CAD build for the part. Positions are in the model's coordinates, mm. A direction names the side the tool comes from. Coordinates: 2 decimals unless noted, no trailing zeros. Loops run counter-clockwise (first coordinate to the right, second up) from the corner with the lowest first, then second, coordinate; pieces in that order, holes last. Notation, with made-up numbers: (18, 83.5) -> (63, 83.5) arc R36 ccw to (63, 121.5) -> close; hole circle Ø1 at (40, -38.75). An arc over 180 degrees is marked (long way). Return JSON: item names as keys, results as strings. Group by question number.
(1) Tool access for faces 4 (the face through (-8.116, -2.521, -4.541)), 5 (the face through (-8.021, -0.014, -9.833)), 6 (the face through (-7, 4, -8.25)): list every direction of +Z, -Z, +X, -X, +Y, -Y with a clear straight run to the whole face (end or side of a thin tool).
(2) Saw through at D-D on y = -2.75. Write the cut outline in (x, z).
(3) Saw through at A-A on y = -4.5. Write the cut outline in (x, z).
(4) Flat gauge pins, fed straight in: pin 1 Ø1.6 at (y, z) = (4.5, -1.5) entering from -X; pin 2 Ø8 at (x, y) = (9.5, -3) entering from -Z; pin 3 Ø1 at (y, z) = (-7.5, -17) entering from +X. Where does each tip first touch, or does it go through?
(5) Saw through at C-C on x = 14. Write the cut outline in (y, z), then the cut area to 3 significant figures.
(6) Probe L1, parallel to Y at x = -8.75, z = -10.75; L2, parallel to Z at x = -3, y = -1.5; L3, parallel to Y at x = -9.5, z = -5.5. List the from-to ranges inside material, lowest first.
(7) Saw through at B-B on y = 1.5. Write the cut outline in (x, z), then the cut area to 3 significant figures.
(8) Mould opens along Y. For faces 1 (the face through (-6, 3, -18)), 2 (the face through (-8.021, -5.014, -9.833)), 3 (the face through (3, 5, -9)) say: pulls with the +Y half, pulls with the -Y half, needs draft (parallel to the pull), parting line crosses it, or undercut.
```python
from build123d import *
from build123d.topology import SkipClean

# Parameters (mm, degrees)
SKETCH1_R           = 1.5
BOSS_EXTRUDE1_DEPTH = 5
BOSS_EXTRUDE2_START = 10
SKETCH2_R           = 1.5
BOSS_EXTRUDE2_DEPTH = 10
CUT_EXTRUDE1_DEPTH  = 2
SKETCH4_OUTSIDE_W   = 39.104
SKETCH4_OUTSIDE_H   = 31.904
SKETCH4_OUTSIDE_R   = 4
CUT_EXTRUDE2_DEPTH  = 2
FILLET4_R           = 7
CUT_EXTRUDE5_START  = -9
CUT_EXTRUDE5_DEPTH  = 7
CUT_EXTRUDE7_START  = 2
CUT_EXTRUDE7_DEPTH  = 2
LPATTERN1_COUNT     = 2
LPATTERN1_PITCH     = 5
CUT_EXTRUDE9_START  = -2
CUT_EXTRUDE9_DEPTH  = 2
LPATTERN2_COUNT     = 2
LPATTERN2_PITCH     = 5
FILLET5_START       = -6
FILLET5_DEPTH       = 2
FILLET5_START_2     = -1
FILLET5_2_DEPTH     = 1


with BuildPart() as part:
    # Sketch1 → Boss-Extrude1 (new body)
    with BuildSketch(Plane(origin=(0, 0, 0), x_dir=(1, 0, 0), z_dir=(0, 1, 0))):
        with BuildLine():
            Line((-12, 14), (-12, 22))
            Line((-12, 22), (-6, 22))
            Line((-6, 22), (-6, 14))
            Line((-6, 14), (0.894304297, 14))
            Line((0.894304297, 14), (6.85307226, 9))
            Line((6.85307226, 9), (11.887670047, 15))
            Line((11.887670047, 15), (15.887670047, 15))
            Line((15.887670047, 15), (17.2, 0))
            Line((17.2, 0), (-3, 0))
            ThreePointArc((-3, 0), (-4.264911064, 0.205266808), (-5.4, 0.8))
            ThreePointArc((-5.4, 0.8), (-10.258048651, 6.620975674), (-12, 14))
        make_face()
        with Locations(Location((-3, 4, 0), (0, 0, 270))):
            Circle(SKETCH1_R, mode=Mode.SUBTRACT)
    extrude(amount=BOSS_EXTRUDE1_DEPTH)

    # Sketch2 → Boss-Extrude2 (add)
    with SkipClean():  # the faces are left unmerged after this step: merging them gives an invalid solid
        with BuildSketch(Plane.XZ.offset(BOSS_EXTRUDE2_START)):
            with BuildLine():
                Line((-12, -14), (-12, -22))
                Line((-12, -22), (-6, -22))
                Line((-6, -22), (-6, -8))
                Line((-6, -8), (-3, -8))
                ThreePointArc((-3, -8), (1, -4), (-3, 0))
                ThreePointArc((-3, 0), (-4.264911064, -0.205266808), (-5.4, -0.8))
                ThreePointArc((-5.4, -0.8), (-10.258048651, -6.620975674), (-12, -14))
            make_face()
            with Locations(Location((-3, -4, 0), (0, 0, 270))):
                Circle(SKETCH2_R, mode=Mode.SUBTRACT)
        extrude(amount=-BOSS_EXTRUDE2_DEPTH)

    # Sketch3 → Cut-Extrude1 (cut)
    with SkipClean():  # the faces are left unmerged after this step: merging them gives an invalid solid
        with BuildSketch(Plane(origin=(0, 5, 0), x_dir=(1, 0, 0), z_dir=(0, 1, 0))):
            with BuildLine():
                Line((1.25, 4), (1.25, 0))
                Line((1.25, 0), (-10.965687828, 0))
                Line((-10.965687828, 0), (-10.965687828, 8.25))
                Line((-10.965687828, 8.25), (-3, 8.25))
                ThreePointArc((-3, 8.25), (0.00520382, 7.00520382), (1.25, 4))
            make_face()
        extrude(amount=-CUT_EXTRUDE1_DEPTH, mode=Mode.SUBTRACT)

    # Sketch4 outside → Cut-Extrude2 (cut)
    with SkipClean():  # the faces are left unmerged after this step: merging them gives an invalid solid
        with BuildSketch(Plane.XZ.offset(10)):
            with Locations((2.6, -11)):
                Rectangle(SKETCH4_OUTSIDE_W, SKETCH4_OUTSIDE_H)
            with Locations(Location((-3, -4, 0), (0, 0, 270))):
                Circle(SKETCH4_OUTSIDE_R, mode=Mode.SUBTRACT)
        extrude(amount=-CUT_EXTRUDE2_DEPTH, mode=Mode.SUBTRACT)

    # Fillet4
    # the kernel refuses this fillet: 7 mm, written as the material it adds along each edge
    with BuildSketch(Plane(origin=(-6, -8, -8), x_dir=(0, 0, -1), z_dir=(0, 1, 0))) as fillet4_piece_1:
        with BuildLine():
            CenterArc((5.744562647, -7), FILLET4_R, 90, 55.150095421)
            Line((0, -3), (0, 0))
            Line((0, 0), (5.744562647, 0))
        make_face()
    extrude(amount=8)

    # Sketch8 → Cut-Extrude5 (cut)
    with BuildSketch(Plane(origin=(0, 3, 0), x_dir=(1, 0, 0), z_dir=(0, 1, 0)).offset(CUT_EXTRUDE5_START)):
        with BuildLine():
            Line((-8.638425733, 4.018428517), (-7.577765561, 5.079088689))
            ThreePointArc((-7.577765561, 5.079088689), (-7.976368998, 5.645642084), (-8.348417241, 6.229977223))
            ThreePointArc((-8.348417241, 6.229977223), (-8.003073705, 8.1765706), (-6.027976147, 8.090097651))
            ThreePointArc((-6.027976147, 8.090097651), (-5.292329992, 7.335150748), (-4.61146284, 6.530452037))
            ThreePointArc((-4.61146284, 6.530452037), (-5.795929923, 5.087554995), (-5.897777479, 3.223542865))
            Line((-5.897777479, 3.223542865), (-6.976385628, 2.144934715))
            ThreePointArc((-6.976385628, 2.144934715), (-7.843003254, 3.050101797), (-8.638425733, 4.018428517))
        make_face()
    extrude(amount=CUT_EXTRUDE5_DEPTH, mode=Mode.SUBTRACT)

    # Sketch10 → Cut-Extrude7 (cut)
    with BuildSketch(Plane.XZ.offset(-1).offset(CUT_EXTRUDE7_START)):
        with BuildLine():
            Line((-8.638425733, -4.018428517), (-7.577765561, -5.079088689))
            Line((-7.577765561, -5.079088689), (-8.348417241, -6.229977223))
            ThreePointArc((-8.348417241, -6.229977223), (-8.556847764, -7.161149711), (-8.16150889, -8.029615404))
            Line((-8.16150889, -8.029615404), (-9.977158514, -6.084074194))
            ThreePointArc((-9.977158514, -6.084074194), (-9.346365817, -5.026251972), (-8.638425733, -4.018428517))
        make_face()
    cut_extrude7 = extrude(amount=-CUT_EXTRUDE7_DEPTH, mode=Mode.SUBTRACT)

    # LPattern1: Cut-Extrude7 ×2
    with Locations(*[(0, -i * LPATTERN1_PITCH, 0) for i in range(1, LPATTERN1_COUNT)]):
        add(cut_extrude7, mode=Mode.SUBTRACT)

    # Sketch11 → Cut-Extrude9 (cut)
    with BuildSketch(Plane.XZ.offset(8).offset(CUT_EXTRUDE9_START)):
        with BuildLine():
            Line((-12, -22), (-6, -22))
            Line((-6, -22), (-6, -11))
            Line((-6, -11), (-10.09871087, -8.633608176))
            ThreePointArc((-10.09871087, -8.633608176), (-9.7258799, -7.711529492), (-9.294878189, -6.815164858))
            Line((-9.294878189, -6.815164858), (-9.977158514, -6.084074194))
            ThreePointArc((-9.977158514, -6.084074194), (-11.486292808, -9.914851011), (-12, -14))
            Line((-12, -14), (-12, -22))
        make_face()
    cut_extrude9 = extrude(amount=-CUT_EXTRUDE9_DEPTH, mode=Mode.SUBTRACT)

    # LPattern2: Cut-Extrude9 ×2
    with Locations(*[(0, i * LPATTERN2_PITCH, 0) for i in range(1, LPATTERN2_COUNT)]):
        add(cut_extrude9, mode=Mode.SUBTRACT)

    # Fillet5: read off the stored shape, not the designer's step
    # Fillet5 outline → Fillet5 (cut)
    with BuildSketch(Plane(origin=(0, 0, 0), x_dir=(1, 0, 0), z_dir=(0, 1, 0)).offset(FILLET5_START)):
        with BuildLine():
            Line((-6, 13.744562647), (-6, 11))
            ThreePointArc((-6, 11), (-5.384425539, 10.558219215), (-4.899169706, 9.976300875))
            ThreePointArc((-4.899169706, 9.976300875), (-5.719158725, 11.781680575), (-6, 13.744562647))
        make_face()
    extrude(amount=FILLET5_DEPTH, mode=Mode.SUBTRACT)

    # Fillet5 2 outline → Fillet5 2 (cut)
    with BuildSketch(Plane(origin=(0, 0, 0), x_dir=(1, 0, 0), z_dir=(0, 1, 0)).offset(FILLET5_START_2)):
        with BuildLine():
            Line((-6, 13.744562647), (-6, 11))
            ThreePointArc((-6, 11), (-5.384425539, 10.558219215), (-4.899169706, 9.976300875))
            ThreePointArc((-4.899169706, 9.976300875), (-5.719158725, 11.781680575), (-6, 13.744562647))
        make_face()
    extrude(amount=FILLET5_2_DEPTH, mode=Mode.SUBTRACT)


solid = part.part
```
Geometry results:
{
 "1": {"face 4": "+Z", "face 5": "-Z, -X", "face 6": "+Z, -X, +Y"},
 "2": {"outline": "(-12, -22) -> (-6, -22) -> (-6, -13.74) arc R7 cw to (-3, -8) arc R4 ccw (long way) to (-5.4, -0.8) arc R16.5 ccw to (-6.98, -2.14) -> (-5.9, -3.22) arc R3 ccw to (-4.61, -6.53) arc R15.02 cw to (-6.03, -8.09) arc R1.5 cw to (-8.35, -6.23) arc R15.02 cw to (-7.58, -5.08) -> (-8.64, -4.02) arc R16.5 ccw to (-12, -14) -> close; hole circle Ø3 at (-3, -4)"},
 "3": {"outline": "(-10.1, -8.63) -> (-6, -11) arc R3 ccw to (-4.9, -9.98) arc R7 cw to (-3, -8) arc R4 ccw (long way) to (-5.4, -0.8) arc R16.5 ccw to (-6.98, -2.14) -> (-5.9, -3.22) arc R3 ccw to (-4.61, -6.53) arc R15.02 cw to (-6.03, -8.09) arc R1.5 cw to (-8.16, -8.03) -> (-9.29, -6.82) arc R15.55 ccw to start; hole circle Ø3 at (-3, -4)"},
 "4": {"pin 1": "x = 1.25", "pin 2": "z = -15", "pin 3": "x = -6"},
 "5": {"outline": "(0, -15) -> (5, -15) -> (5, 0) -> (0, 0) -> close", "area": "75.0 mm²"},
 "6": {"L1": "-8 to -6, -4 to -1, 1 to 5", "L2": "-8 to -5.5, -2.5 to 0", "L3": "-8 to -6, -4 to -1, 1 to 3"},
 "7": {"outline": "(-12, -22) -> (-6, -22) -> (-6, -14) -> (0.89, -14) -> (6.85, -9) -> (11.89, -15) -> (15.89, -15) -> (17.2, 0) -> (-3, 0) arc R4 ccw to (-5.4, -0.8) arc R16.5 ccw to (-12, -14) -> close; hole circle Ø3 at (-3, -4)", "area": "388 mm²"},
 "8": {"face 1": "needs draft", "face 2": "undercut", "face 3": "pulls with the +Y half"}
}
